Could you check a few things on this model? Use its own coordinates, in mm. A direction names the side the tool comes from. Give positions to 0.01 mm unless a question says otherwise; leave off trailing zeros. Loops run counter-clockwise (first coordinate to the right, second up) from the corner with the lowest first, then second, coordinate; pieces in that order, holes last. Notation, with made-up numbers: M 19.25,-14.75 L 34.25,-14.75 A21 ccw 34.25,-2.75 Z; hole C 52,16 d7. An arc over 180 degrees is marked long. Write each question's results on one line, items separated by ' | '. Start each with the question number.
from build123d import *

# Parameters (mm, degrees)
EXTRUDE1_DEPTH     = 17.78
EXTRUDE1_DRAFT     = 5
SKETCH3_R          = 4.445
CUT_EXTRUDE2_DEPTH = 18.78
CUT_EXTRUDE3_DEPTH = 18.78
CUT_EXTRUDE3_TAPER = 5
SKETCH5_R          = 10.522638874
CUT_EXTRUDE4_DEPTH = 26.162
SKETCH6_R          = 3.2639
CUT_EXTRUDE5_DEPTH = 7.62


with BuildPart() as part:
    # Sketch1 → Extrude1 (with draft: the straight prism first)
    with BuildSketch(Plane.XY):
        with BuildLine():
            ThreePointArc((-195.012025381, 26.062859944), (-204.895443331, 2.202178287), (-195.012025381, -21.658503371))
            Line((-195.012025381, -21.658503371), (-195.012025381, -36.94271364))
            ThreePointArc((-195.012025381, -36.94271364), (-195.978739559, -54.984528068), (-177.936925131, -54.017813891))
            Line((-177.936925131, -54.017813891), (-134.591688961, -54.017813891))
            ThreePointArc((-134.591688961, -54.017813891), (-120.832429722, 2.202178287), (-134.591688961, 58.422170464))
            Line((-134.591688961, 58.422170464), (-177.936925131, 58.422170464))
            ThreePointArc((-177.936925131, 58.422170464), (-195.978739559, 59.388884642), (-195.012025381, 41.347070214))
            Line((-195.012025381, 41.347070214), (-195.012025381, 26.062859944))
        make_face()
    extrude(amount=EXTRUDE1_DEPTH)
    # Extrude1: the draft: its side faces are tilted about the plane it starts from
    extrude1_sides = [part.faces().sort_by_distance(p)[0] for p in [
        (-204.895443331, 2.202178287, 8.89),
        (-195.012025381, -29.300608506, 8.89),
        (-195.978739559, -54.984528068, 8.89),
        (-156.264307046, -54.017813891, 8.89),
        (-120.832429722, 2.202178287, 8.89),
        (-156.264307046, 58.422170464, 8.89),
        (-195.978739559, 59.388884642, 8.89),
        (-195.012025381, 33.704965079, 8.89),
    ]]
    draft(extrude1_sides, Plane.XY, EXTRUDE1_DRAFT)

    # Sketch3 → Cut-Extrude2 (cut, through all)
    with BuildSketch(Plane(origin=(10.378673568, 21.507111235, 17.78), x_dir=(1, 0, 0), z_dir=(0, 0, 1))):
        with Locations((-197.770698949, 29.295059229)):
            Circle(SKETCH3_R)
        with Locations((-197.770698949, -67.904925126)):
            Circle(SKETCH3_R)
    extrude(amount=-CUT_EXTRUDE2_DEPTH, mode=Mode.SUBTRACT)

    # Sketch4 → Cut-Extrude3 (cut, through all)
    with BuildSketch(Plane.XY.offset(17.78)):
        with BuildLine():
            ThreePointArc((-177.936489958, 26.267275972), (-196.154686221, 2.202178287), (-177.936489958, -21.862919399))
            ThreePointArc((-177.936489958, -21.862919399), (-172.405947357, -21.316646023), (-168.71726973, -17.159847564))
            ThreePointArc((-168.71726973, -17.159847564), (-165.268623085, 2.202178287), (-168.71726973, 21.564204137))
            ThreePointArc((-168.71726973, 21.564204137), (-172.405947357, 25.721002597), (-177.936489958, 26.267275972))
        make_face()
    extrude(amount=-CUT_EXTRUDE3_DEPTH, taper=CUT_EXTRUDE3_TAPER, mode=Mode.SUBTRACT)

    # Sketch5 → Cut-Extrude4 (cut)
    with BuildSketch(Plane(origin=(0, 0, 0), x_dir=(-1, 0, 0), z_dir=(0, 0, -1))):
        with Locations((134.591688961, 58.422170464)):
            Circle(SKETCH5_R)
        with Locations((134.591688961, -54.017813891)):
            Circle(SKETCH5_R)
    extrude(amount=-CUT_EXTRUDE4_DEPTH, mode=Mode.SUBTRACT)

    # Sketch6 → Cut-Extrude5 (cut)
    with BuildSketch(Plane.XY.offset(17.78)):
        with Locations((-162.563054604, 44.430433633)):
            Circle(SKETCH6_R)
        with Locations((-162.563054604, -40.394882783)):
            Circle(SKETCH6_R)
    extrude(amount=-CUT_EXTRUDE5_DEPTH, mode=Mode.SUBTRACT)


solid = part.part
1) Which directions (+Z, -Z, +X, -X, +Y, -Y) give clear straight access to the entire face, cutting with the end or side of a thin tool? Please do faces 5 (the face through (-194.245, 33.883, 8.766)), 6 (the face through (-162.09, -53.25, 8.77)), 7 (the face through (-161.62, 57.655, 8.766)), 8 (the face through (-161.057, 41.535, 14.023)).
2) If we section it at B-B on z = 7: State how many separate pieces and enclosed holes the cut face has, plus the area to 3 significant figures.
3) I'm going to push flat-ended pins straight in: P1, Ø3.5, axis at x = -163, y = 45, coming from the +Z side; P2, Ø10, axis at x = -160.5, z = 4, coming from the -Y side; P3, Ø8, axis at x = -188, z = 7.5, coming from the -Y side. Where does each tip first touch, or does it pass through?
4) Thinking about a two-plate mould opening in Y: for faces 1 (the face through (-163, 3, 0)), 2 (the face through (-140.12, 49.47, 8.77)), 3 (the face through (-140.368, -45.222, 8.766)), 4 (the face through (-163, -40, 10.16)), which applies, pulls with the +Y half, pulls with the -Y half, needs draft (parallel to the pull), parting line crosses it, or undercut?
5) If we section it at D-D on x = -136: Write out the boundary of the cut face in (y, z), plus the area to 3 significant figures.
6) Please list where these lines run through material, in increasing order: line 1 (Y direction, x = -190, z = 13.25); line 2 (X direction, y = 17, z = 11.5); line 3 (X direction, y = 21.5, z = 7). Write a range as from..to.
7) If we section it at A-A on x = -149: Write out the boundary of the cut face in (y, z), plus the area to 3 significant figures.
Calculated:
1) face 5: +Z, -X | face 6: +Z, +X, -Y | face 7: +Z, +X, +Y | face 8: +Z
2) separate pieces: 1 | enclosed holes: 3 | area: 6,800 mm2
3) P1: stops at z = 10.16 | P2: stops at y = -54.02 | P3: stops at y = -58.23
4) face 1: needs draft | face 2: pulls with the +Y half | face 3: pulls with the -Y half | face 4: undercut
5) outline: M -43.59,0 L 47.99,0 L 47.99,17.78 L -43.59,17.78 Z | area: 1,630 mm2
6) line 1: y = -57.07..-50, -42.8..-13.62, 18.02..47.2, 54.4..61.47 | line 2: x = -200.35..-190.62, -167.83..-122.75 | line 3: x = -198.08..-185.52, -169.7..-122.99
7) outline: M -54.02,0 L 58.42,0 L 56.87,17.78 L -52.46,17.78 Z | area: 1,970 mm2
